from build123d import *
from build123d.topology import SkipClean

# Parameters (mm, degrees)
SKETCH3_R               = 10
SKETCH3_R_2             = 6
SKETCH7_R               = 2
CUT_EXTRUDE1_DEPTH      = 89.834115151
CIRPATTERN1_COUNT       = 4
MIRROR2_COPY_1_SKETCH_R = 2
MIRROR2_COPY_1_DEPTH    = 89.834115151
MIRROR2_COPY_2_SKETCH_R = 2
MIRROR2_COPY_2_DEPTH    = 89.834115151
MIRROR2_COPY_3_SKETCH_R = 2
MIRROR2_COPY_3_DEPTH    = 89.834115151


with BuildPart() as part:
    # Sweep-Thin2: sweep along a path in Sketch1
    with BuildLine(Plane.XY) as sweep_thin2_path:
        Line((-30, -33), (-30, 0))
        ThreePointArc((-30, 0), (0, 30), (30, 0))
        Line((30, 0), (30, -33))
    # Sketch3 → Sweep-Thin2 (sweep)
    with BuildSketch(Plane(origin=(0, -33, 0), x_dir=(1, 0, 0), z_dir=(0, 1, 0))):
        with Locations((-30, 0)):
            Circle(SKETCH3_R)
        with Locations((-30, 0)):
            Circle(SKETCH3_R_2, mode=Mode.SUBTRACT)
    sweep(path=sweep_thin2_path.line)

    # Sketch4 → Revolve2 (revolve)
    with SkipClean():  # the faces are left unmerged after this step: merging them gives an invalid solid
        with BuildSketch(Plane.XY, mode=Mode.PRIVATE) as revolve2_sk:
            Polygon((36, -33), (47.5, -33), (47.5, -34.2), (46.3, -34.2), (46.3, -38.8), (47.5, -38.8), (47.5, -40), (36, -40), align=None)
        revolve2 = revolve(revolve2_sk.sketch.rotate(Axis((30, -33, 0), (0, -1, 0)), 90), axis=Axis((30, -33, 0), (0, -1, 0)))
    add(part.part.scale(1), mode=Mode.REPLACE)  # the faces are merged on a copy

    # Sketch7 → Cut-Extrude1 (cut, through all)
    with BuildSketch(Plane(origin=(0, -33, 0), x_dir=(1, 0, 0), z_dir=(0, 1, 0))):
        with Locations(Location((43.614766478, 0, 0), (0, 0, 270))):
            Circle(SKETCH7_R)
    cut_extrude1 = extrude(amount=-CUT_EXTRUDE1_DEPTH, mode=Mode.SUBTRACT)

    # CirPattern1: Cut-Extrude1 ×4 about axis
    cirpattern1_axis = Axis((30, 0, 0), (0, 1, 0))
    for i in range(1, CIRPATTERN1_COUNT):
        add(cut_extrude1.rotate(cirpattern1_axis, i * 360 / CIRPATTERN1_COUNT), mode=Mode.SUBTRACT)

    # Mirror2: Revolve2, Cut-Extrude1 across plane
    with SkipClean():  # the faces are left unmerged after this step: merging them gives an invalid solid
        add(revolve2.mirror(Plane(origin=(0, 0, 0), x_dir=(0, 0, 1), z_dir=(1, 0, 0))))
        add(cut_extrude1.mirror(Plane(origin=(0, 0, 0), x_dir=(0, 0, 1), z_dir=(1, 0, 0))), mode=Mode.SUBTRACT)

    # Mirror2 copy 1 sketch → Mirror2 copy 1 (cut, through all)
    with SkipClean():  # the faces are left unmerged after this step: merging them gives an invalid solid
        with BuildSketch(Plane(origin=(-30, -33, 30), x_dir=(0, 0, -1), z_dir=(0, 1, 0))):
            with Locations((43.614766478, 0)):
                Circle(MIRROR2_COPY_1_SKETCH_R)
        extrude(amount=-MIRROR2_COPY_1_DEPTH, mode=Mode.SUBTRACT)

    # Mirror2 copy 2 sketch → Mirror2 copy 2 (cut, through all)
    with SkipClean():  # the faces are left unmerged after this step: merging them gives an invalid solid
        with BuildSketch(Plane(origin=(-60, -33, 0), x_dir=(1, 0, 0), z_dir=(0, 1, 0))):
            with Locations((43.614766478, 0)):
                Circle(MIRROR2_COPY_2_SKETCH_R)
        extrude(amount=-MIRROR2_COPY_2_DEPTH, mode=Mode.SUBTRACT)

    # Mirror2 copy 3 sketch → Mirror2 copy 3 (cut, through all)
    with SkipClean():  # the faces are left unmerged after this step: merging them gives an invalid solid
        with BuildSketch(Plane(origin=(-30, -33, -30), x_dir=(0, 0, 1), z_dir=(0, 1, 0))):
            with Locations((43.614766478, 0)):
                Circle(MIRROR2_COPY_3_SKETCH_R)
        extrude(amount=-MIRROR2_COPY_3_DEPTH, mode=Mode.SUBTRACT)


solid = part.part
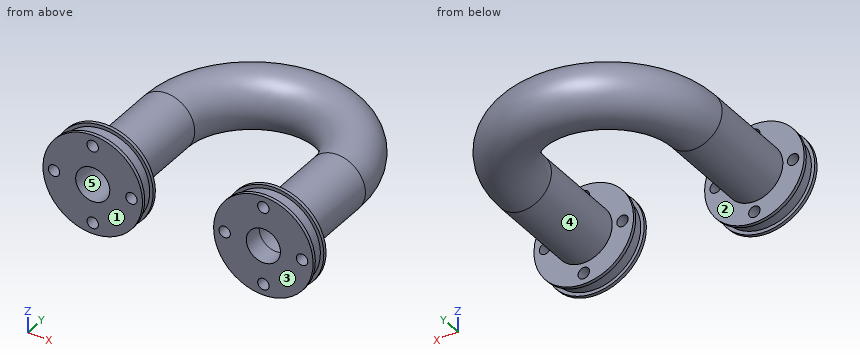
Part model, mm, in its own coordinate system. Face numbers are marked on the shaded views. A direction names the side the tool comes from. Round coordinates to 2 decimals unless told otherwise and drop trailing zeros. Loops run counter-clockwise (first coordinate to the right, second up) from the corner with the lowest first, then second, coordinate; pieces in that order, holes last. Notation, with made-up numbers: (-39, 7) - (-30, 7) arc R12 cw to (-30, 13) - close; hole circle Ø8 at (75, -16). An arc over 180 degrees is marked (long way). Answer as a JSON object with one key per item and string values.
Item 1: Band-saw the part on B-B on x = -30. State how many separate pieces and enclosed holes the cut face has, plus the area to 3 significant figures.
Output:
{"separate pieces": "3", "enclosed holes": "0", "area": "607 mm2"}
Item 2: Tool access for the marked faces 1 and 2: list every direction of +Z, -Z, +X, -X, +Y, -Y with a clear straight run to the whole face (end or side of a thin tool).
Output:
{"face 1": "+Z, -Z, +X, -X, -Y", "face 2": "none"}
Item 3: Pin check, flat tips, straight feed: pin 1 (8 mm diameter, centred on y = -13.5, z = 6.5, fed in from -X); pin 2 (4.5 mm diameter, centred on x = 16.39, z = 0, fed in from +Y); pin 3 (17.5 mm diameter, centred on x = 23.5, z = 0.5, fed in from +Y). Stop position of each tip, or through.
Output:
{"pin 1": "x = -39.68", "pin 2": "y = 37.42", "pin 3": "y = 37.18"}
Item 4: Wall check: L1, parallel to Z at x = 30, y = -36.5; L2, parallel to X at y = -31, z = 2.5; L3, parallel to Z at x = -30, y = -28.5. Give the ranges that are in metal, low to high.
Output:
{"L1": "-16.3 to -15.61, -11.61 to -6, 6 to 11.61, 15.61 to 16.3", "L2": "-39.68 to -35.45, -24.55 to -20.32, 20.32 to 24.55, 35.45 to 39.68", "L3": "-10 to -6, 6 to 10"}
Item 5: Pull direction Y, two halves, no side cores. Call the marked faces 3, 4 and 5: pulls with the +Y half, pulls with the -Y half, needs draft (parallel to the pull), parting line crosses it, or undercut.
Output:
{"face 3": "pulls with the -Y half", "face 4": "undercut", "face 5": "needs draft"}
Item 6: Band-saw the part on A-A on y = -31. List the corners of the cut face in (x, z).
Output:
{"outline": "circle Ø20 at (-30, 0); circle Ø20 at (30, 0); hole circle Ø12 at (-30, 0); hole circle Ø12 at (30, 0)"}
